```python
from build123d import *

# Parameters (mm, degrees)
SKETCH1_W           = 31
SKETCH1_H           = 14.3
BOSS_EXTRUDE1_DEPTH = 1.5
SKETCH2_W           = 0.5
SKETCH2_H           = 4
BOSS_EXTRUDE2_DEPTH = 14.3
SKETCH5_R           = 1.5
CUT_EXTRUDE1_DEPTH  = 1.5


with BuildPart() as part:
    # Sketch1 → Boss-Extrude1 (new body)
    with BuildSketch(Plane.XY):
        with Locations((15.5, 0)):
            Rectangle(SKETCH1_W, SKETCH1_H)
    extrude(amount=BOSS_EXTRUDE1_DEPTH)

    # Sketch2 → Boss-Extrude2 (add, through all)
    with BuildSketch(Plane.XZ.offset(7.15)):
        with Locations((2.25, 3.5)):
            Rectangle(SKETCH2_W, SKETCH2_H)
    extrude(amount=-BOSS_EXTRUDE2_DEPTH)

    # Sketch4 → Revolve1 (revolve)
    with BuildSketch(Plane.XZ.offset(3.15)):
        with BuildLine():
            Line((2.25, 14), (2.25, 5.5))
            Line((2.25, 5.5), (5.05, 5.5))
            Line((5.05, 5.5), (5.05, 6.5))
            Line((5.05, 6.5), (4.75, 6.5))
            Line((4.75, 6.5), (4.75, 11.499998492))
            ThreePointArc((4.75, 11.499998492), (4.017767486, 13.26776642), (2.25, 14))
        make_face()
    revolve1 = revolve(axis=Axis((2.25, -3.15, 14), (0, 0, -1)))

    # Mirror1: Revolve1 across plane
    add(revolve1.mirror(Plane.ZX))

    # Sketch5 → Cut-Extrude1 (cut)
    with BuildSketch(Plane.XY.offset(1.5)):
        with Locations((25.5, 0)):
            Circle(SKETCH5_R)
    extrude(amount=-CUT_EXTRUDE1_DEPTH, mode=Mode.SUBTRACT)


solid = part.part
```
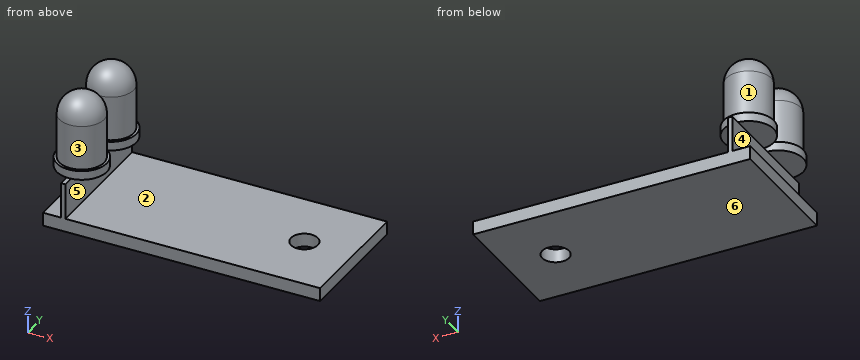
Here's how the part is built. I have some questions about the finished solid (model axes, mm). Face numbers are marked on the shaded views. A direction names the side the tool comes from. Give positions to 0.01 mm unless a question says otherwise; leave off trailing zeros. Write each loop counter-clockwise with the first axis right and the second up, starting at its lowest first coordinate (ties: lowest second). Pieces come first, ordered by that corner, then holes. Notation, with made-up numbers: (55.25, 38.5) -> (77.25, 38.5) arc R20 ccw to (77.25, 43.5) -> close; hole circle Ø2 at (38.25, -18.75). An arc over 180 degrees is marked (long way). Use one line per item in the form item = value.
1) Suppose I cut it at C-C (z = 8.5). Please give me the cut outline in (x, y), and give its area (3 significant figures).
Verdict:
outline = circle Ø5 at (2.25, -3.15); circle Ø5 at (2.25, 3.15)
area = 39.3 mm2
2) On a 3-axis mill with a long thin cutter (end or side, diameter ignored), from which of +Z, -Z, +X, -X, +Y, -Y can I reach the whole of each face in a straight line? I mean the marked faces 4, 5 and 6. Say none if no direction works.
Verdict:
face_4 = -X, +Y, -Y
face_5 = +X, +Y, -Y
face_6 = -Z, +X, -X, +Y, -Y
3) I'm going to push flat-ended pins straight in: pin 1 (1.6 mm diameter, centred on x = 1, y = -1.5, fed in from +Z); pin 2 (2.5 mm diameter, centred on x = 25.5, y = 0, fed in from +Z); pin 3 (3 mm diameter, centred on x = 17.5, y = -2, fed in from +Z); pin 4 (0.6 mm diameter, centred on x = 2, y = 0, fed in from +Z). Where does each tip first touch, or does it pass through?
Verdict:
pin_1 = 13.65
pin_2 = through
pin_3 = 1.5
pin_4 = 5.5
4) We'd pull the mould along Y, two halves only. Please class the marked faces 1, 2 and 3: +Y half, -Y half, draft (parallel to the pull), parting line (faces both ways), or undercut.
Verdict:
face_1 = undercut
face_2 = draft
face_3 = undercut
5) Suppose I cut it at D-D (x = 3). Please give me the cut outline in (y, z).
Verdict:
outline = (-7.15, 0) -> (7.15, 0) -> (7.15, 1.5) -> (-7.15, 1.5) -> close; (-5.85, 5.5) -> (-0.45, 5.5) -> (-0.45, 6.5) -> (-0.77, 6.5) -> (-0.77, 11.5) arc R2.38 ccw to (-5.53, 11.5) -> (-5.53, 6.5) -> (-5.85, 6.5) -> close; (0.45, 5.5) -> (5.85, 5.5) -> (5.85, 6.5) -> (5.53, 6.5) -> (5.53, 11.5) arc R2.38 ccw to (0.77, 11.5) -> (0.77, 6.5) -> (0.45, 6.5) -> close
6) Suppose I cut it at B-B (y = 0). Please give me the cut outline in (x, z), and give its area (3 significant figures).
Verdict:
outline = (0, 0) -> (24, 0) -> (24, 1.5) -> (2.5, 1.5) -> (2.5, 5.5) -> (2, 5.5) -> (2, 1.5) -> (0, 1.5) -> close; (27, 0) -> (31, 0) -> (31, 1.5) -> (27, 1.5) -> close
area = 44.0 mm2
7) If I drill on L1, parallel to Y at x = 25.5, z = 0.9; L2, parallel to Z at x = 5.5, y = -4.75; L3, parallel to X at y = -0.5, z = 4.25, over which ranges is the centre line in solid material (lowest first)? Write a range as [from, to].
Verdict:
L1 = [-7.15, -1.5], [1.5, 7.15]
L2 = [0, 1.5]
L3 = [2, 2.5]
8) Suppose I cut it at A-A (x = 25.5). Please give me the cut outline in (y, z), and give its area (4 significant figures).
Verdict:
outline = (-7.15, 0) -> (-1.5, 0) -> (-1.5, 1.5) -> (-7.15, 1.5) -> close; (1.5, 0) -> (7.15, 0) -> (7.15, 1.5) -> (1.5, 1.5) -> close
area = 16.95 mm2
